Autodesk Fusion 360 part; units mm, degrees
sketch "Sketch1" plane through (0, 0, 0) normal (0, 0, 1) x (1, 0, 0)
  line L0 (33.4251, -19.298) -> (33.4251, 19.298)
  line L1 (33.4251, 19.298) -> (0, 38.596)
  line L2 (0, 38.596) -> (-33.4251, 19.298)
  line L3 (-33.4251, 19.298) -> (-33.4251, -19.298)
  line L4 (-33.4251, -19.298) -> (0, -38.596)
  line L5 (0, -38.596) -> (33.4251, -19.298)
  dimension "d1" = 38.596
extrude "Extrude1" add sketch "Sketch1" along normal blind 2.5
sketch "Sketch2" plane through (0, 0, 2.5) normal (0, 0, 1) x (-1, 0, 0)
  line L0 (0, 38.596) -> (-33.4251, 19.298)
  line L1 (-33.4251, 19.298) -> (-33.4251, -19.298)
  line L2 (-33.4251, -19.298) -> (0, -38.596)
  line L3 (0, -38.596) -> (33.4251, -19.298)
  line L4 (33.4251, -19.298) -> (33.4251, 19.298)
  line L5 (33.4251, 19.298) -> (0, 38.596)
  circle A0 centre (0, 0) radius 16.5
  dimension "d4" = 33
extrude "Extrude2" add sketch "Sketch2" along normal blind 4 draft -45 contours A0
sketch "Sketch3" plane through (0, 0, 6.5) normal (0, 0, 1) x (-1, 0, 0)
  circle A0 centre (0, 0) radius 12.5
  circle A1 centre (0, 0) radius 10
  dimension "d7" = 20
extrude "Extrude3" add sketch "Sketch3" along normal blind 8.5
For this review, take the finished solid that the model builds, in its own axes (mm). A direction names the side the tool comes from. Round coordinates to 2 decimals unless told otherwise and drop trailing zeros. Write each loop counter-clockwise with the first axis right and the second up, starting at its lowest first coordinate (ties: lowest second). Pieces come first, ordered by that corner, then holes. Notation, with made-up numbers: (-26, 35.5) -> (-1, 35.5) arc R25 ccw to (-1, 74.5) -> close; hole circle Ø8 at (13, 84). An arc over 180 degrees is marked (long way). Use one line per item in the form item = value.
1) Take a section at B-B, the plane z = 1.25. Write out the cut boundary in (x, y), and give its area (3 significant figures).
Found:
outline = (-33.43, -19.3) -> (0, -38.6) -> (33.43, -19.3) -> (33.43, 19.3) -> (0, 38.6) -> (-33.43, 19.3) -> close
area = 3,870 mm2
2) Mouldability with a two-part tool opening along Y and no side actions: class faces 3 (the cylindrical face through (2.17, -9.76, 10.69)), 4 (the flat face through (0, -17, 2.5)), 5 (the flat face through (-16.95, -28.81, 1.23)) as +Y half, -Y half, draft (parallel to the pull), parting line (faces both ways), or undercut.
Found:
face_3 = undercut
face_4 = draft
face_5 = -Y half
3) Clearance check with flat-ended pins moving along their axes: pin 1 (16 mm diameter, centred on x = 0, y = 0, fed in from +Z); pin 2 (6 mm diameter, centred on x = -12, y = 30, fed in from +Z); pin 3 (6 mm diameter, centred on x = -24.5, y = -30.5, fed in from -Z); pin 4 (3 mm diameter, centred on x = 7, z = 7, fed in from +Y). State where each tip first meets the part, or that it passes through.
Found:
pin_1 = 6.5
pin_2 = 2.5
pin_3 = through
pin_4 = 11.75
4) To check wall thickness, follow L1, parallel to Y at x = 0, z = 10.25; L2, parallel to Z at x = -14, y = -22. State the ranges of each line that lie inside material, in increasing order. Write a range as from..to.
Found:
L1 = -12.5..-10, 10..12.5
L2 = 0..2.5
5) Tool access review of faces 1 (the cylindrical face through (-11.923, 3.755, 10.69)), 2 (the flat face through (16.95, 28.81, 1.23)): name each direction out of +Z, -Z, +X, -X, +Y, -Y from which nothing blocks a thin tool from reaching the whole face with its end or side.
Found:
face_1 = +Z
face_2 = +Z, -Z, +X, +Y
6) Take a section at D-D, the plane x = -19. Write out the cut boundary in (y, z), and give its area (3 significant figures).
Found:
outline = (-27.63, 0) -> (27.63, 0) -> (27.63, 2.5) -> (-27.63, 2.5) -> close
area = 138 mm2
7) Take a section at C-C, the plane z = 7.75. Write out the cut boundary in (x, y), and give its area (3 significant figures).
Found:
outline = circle Ø25 at (0, 0); hole circle Ø20 at (0, 0)
area = 177 mm2
8) Take a section at A-A, the plane y = 0. Write out the cut boundary in (x, z), and give its area (3 significant figures).
Found:
outline = (-33.43, 0) -> (33.43, 0) -> (33.43, 2.5) -> (16.5, 2.5) -> (12.5, 6.5) -> (12.5, 15) -> (10, 15) -> (10, 6.5) -> (-10, 6.5) -> (-10, 15) -> (-12.5, 15) -> (-12.5, 6.5) -> (-16.5, 2.5) -> (-33.43, 2.5) -> close
area = 326 mm2
